from build123d import *
from build123d.topology import SkipClean

# Parameters (mm, degrees)
SKETCH_2_R               = 4.5
EXTRUDE_1_DEPTH          = 8
EXTRUDE_2_DEPTH          = 4
EXTRUDE_2_DEPTH_BACK     = 11.5
CUT_EXTRUDE_1_DEPTH      = 41.717122437
CUT_EXTRUDE_1_DEPTH_BACK = 41.717122437
CUT_EXTRUDE_2_DEPTH      = 41.717122437
CUT_EXTRUDE_2_DEPTH_BACK = 41.717122437
SKETCH_6_R               = 1
SKETCH_7_R               = 1.75
EXTRUDE_3_DEPTH          = 3
EXTRUDE_4_DEPTH          = 5
SKETCH_9_R               = 1
CUT_EXTRUDE_3_DEPTH      = 5
SKETCH_10_R              = 3.5
SKETCH_10_R_2            = 1
EXTRUDE_5_DEPTH          = 4


with BuildPart() as part:
    # Sketch 2 → Extrude 1 (new body)
    with BuildSketch(Plane.XY):
        with BuildLine():
            Line((-18.858561718, 18.044523082), (33.641438282, 18.044523082))
            ThreePointArc((33.641438282, 18.044523082), (34.348545063, 17.751629864), (34.641438282, 17.044523082))
            Line((34.641438282, 17.044523082), (34.641438282, 7.044523082))
            ThreePointArc((34.641438282, 7.044523082), (34.348545063, 6.337416301), (33.641438282, 6.044523082))
            Line((33.641438282, 6.044523082), (22.641438282, 6.044523082))
            ThreePointArc((22.641438282, 6.044523082), (19.105904376, 4.580056988), (17.641438282, 1.044523082))
            Line((17.641438282, 1.044523082), (17.641438282, -12.955476918))
            ThreePointArc((17.641438282, -12.955476918), (17.348545063, -13.662583699), (16.641438282, -13.955476918))
            Line((16.641438282, -13.955476918), (-9.858561718, -13.955476918))
            ThreePointArc((-9.858561718, -13.955476918), (-10.565668499, -13.662583699), (-10.858561718, -12.955476918))
            Line((-10.858561718, -12.955476918), (-10.858561718, 6.044523082))
            Line((-10.858561718, 6.044523082), (-17.858561718, 6.044523082))
            ThreePointArc((-17.858561718, 6.044523082), (-18.565668499, 6.337416301), (-18.858561718, 7.044523082))
            Line((-18.858561718, 7.044523082), (-18.858561718, 18.044523082))
        make_face()
        with Locations((-0.858561718, -3.955476918)):
            Circle(SKETCH_2_R, mode=Mode.SUBTRACT)
    extrude(amount=EXTRUDE_1_DEPTH)

    # Sketch 3 → Extrude 2 (add, two sides: drawn at the far end of the back side and taken through both)
    with SkipClean():  # the faces are left unmerged after this step: merging them gives an invalid solid
        with BuildSketch(Plane.XY.offset(8).offset(-EXTRUDE_2_DEPTH_BACK)):
            with BuildLine():
                Line((27.141438282, 14.544523082), (27.141438282, 18.044523082))
                Line((27.141438282, 18.044523082), (33.141438282, 18.044523082))
                Line((33.141438282, 18.044523082), (33.141438282, 14.544523082))
                ThreePointArc((33.141438282, 14.544523082), (30.141438282, 11.544523082), (27.141438282, 14.544523082))
            make_face()
            with BuildLine():
                Line((-0.358561718, 14.544523082), (-0.358561718, 18.044523082))
                Line((-0.358561718, 18.044523082), (-6.358561718, 18.044523082))
                Line((-6.358561718, 18.044523082), (-6.358561718, 14.544523082))
                ThreePointArc((-6.358561718, 14.544523082), (-3.358561718, 11.544523082), (-0.358561718, 14.544523082))
            make_face()
            with BuildLine():
                Line((-6.358561718, -10.455476918), (-6.358561718, -13.955476918))
                Line((-6.358561718, -13.955476918), (-0.358561718, -13.955476918))
                Line((-0.358561718, -13.955476918), (-0.358561718, -10.455476918))
                ThreePointArc((-0.358561718, -10.455476918), (-0.519059003, -9.487373446), (-0.983377938, -8.622855294))
                ThreePointArc((-0.983377938, -8.622855294), (-1.135599023, -8.491670945), (-1.327173883, -8.4310107))
                ThreePointArc((-1.327173883, -8.4310107), (-2.473967575, -8.155532145), (-3.509794913, -7.591541073))
                ThreePointArc((-3.509794913, -7.591541073), (-3.692643427, -7.508192328), (-3.893539312, -7.503562458))
                ThreePointArc((-3.893539312, -7.503562458), (-5.661270208, -8.532579726), (-6.358561718, -10.455476918))
            make_face()
        extrude(amount=EXTRUDE_2_DEPTH + EXTRUDE_2_DEPTH_BACK)
    add(part.part.scale(1), mode=Mode.REPLACE)  # the faces are merged on a copy

    # Sketch 5 → Cut-Extrude 1 (cut, two sides: drawn at the far end of the back side and taken through both)
    with BuildSketch(Plane.XY.offset(8).offset(-CUT_EXTRUDE_1_DEPTH_BACK)):
        with BuildLine():
            Line((8.520862779, 6.560547497), (2.520862779, 6.560547497))
            ThreePointArc((2.520862779, 6.560547497), (0.399542436, 5.681867841), (-0.479137221, 3.560547497))
            Line((-0.479137221, 3.560547497), (-0.479137221, -8.439452503))
            Line((-0.479137221, -8.439452503), (8.520862779, -8.439452503))
            ThreePointArc((8.520862779, -8.439452503), (10.642183123, -7.560772847), (11.520862779, -5.439452503))
            Line((11.520862779, -5.439452503), (11.520862779, 3.560547497))
            ThreePointArc((11.520862779, 3.560547497), (10.642183123, 5.681867841), (8.520862779, 6.560547497))
        make_face()
    extrude(amount=CUT_EXTRUDE_1_DEPTH + CUT_EXTRUDE_1_DEPTH_BACK, mode=Mode.SUBTRACT)

    # Sketch 6 → Cut-Extrude 2 (cut, two sides: drawn at the far end of the back side and taken through both)
    with BuildSketch(Plane.XY.offset(8).offset(-CUT_EXTRUDE_2_DEPTH_BACK)):
        with Locations((-3.358561718, 14.544523082)):
            Circle(SKETCH_6_R)
        with Locations((30.141438282, 14.544523082)):
            Circle(SKETCH_6_R)
        with Locations((-3.358561718, -10.455476918)):
            Circle(SKETCH_6_R)
    extrude(amount=CUT_EXTRUDE_2_DEPTH + CUT_EXTRUDE_2_DEPTH_BACK, mode=Mode.SUBTRACT)

    # Sketch 7 → Extrude 3 (add)
    with BuildSketch(Plane(origin=(0, 18.044523082, 0), x_dir=(1, 0, 0), z_dir=(0, 1, 0))):
        with BuildLine():
            Line((-31.858561718, 15.5), (95.141438282, 15.5))
            ThreePointArc((95.141438282, 15.5), (98.656156908, 7.014718626), (107.141438282, 3.5))
            Line((107.141438282, 3.5), (107.141438282, -56.5))
            ThreePointArc((107.141438282, -56.5), (98.656156908, -60.014718626), (95.141438282, -68.5))
            Line((95.141438282, -68.5), (-31.858561718, -68.5))
            ThreePointArc((-31.858561718, -68.5), (-35.373280344, -60.014718626), (-43.858561718, -56.5))
            Line((-43.858561718, -56.5), (-43.858561718, 3.5))
            ThreePointArc((-43.858561718, 3.5), (-35.373280344, 7.014718626), (-31.858561718, 15.5))
        make_face()
        with Locations(Location((-37.858561718, -26.5, 0), (0, 0, 180))):
            Circle(SKETCH_7_R, mode=Mode.SUBTRACT)
        with Locations(Location((-37.858561718, -50, 0), (0, 0, 180))):
            Circle(SKETCH_7_R, mode=Mode.SUBTRACT)
        with Locations(Location((-37.858561718, -3, 0), (0, 0, 180))):
            Circle(SKETCH_7_R, mode=Mode.SUBTRACT)
        with Locations((101.141438282, -50)):
            Circle(SKETCH_7_R, mode=Mode.SUBTRACT)
        with Locations((101.141438282, -26.5)):
            Circle(SKETCH_7_R, mode=Mode.SUBTRACT)
        with Locations((101.141438282, -3)):
            Circle(SKETCH_7_R, mode=Mode.SUBTRACT)
    extrude(amount=EXTRUDE_3_DEPTH)

    # Sketch 8 → Extrude 4 (add)
    with BuildSketch(Plane.XZ.offset(-18.044523082)):
        with BuildLine():
            Line((90.141438282, 31), (44.141438282, 31))
            ThreePointArc((44.141438282, 31), (42.72722472, 30.414213562), (42.141438282, 29))
            Line((42.141438282, 29), (42.141438282, 28))
            ThreePointArc((42.141438282, 28), (42.72722472, 26.585786438), (44.141438282, 26))
            Line((44.141438282, 26), (90.141438282, 26))
            ThreePointArc((90.141438282, 26), (91.555651845, 26.585786438), (92.141438282, 28))
            Line((92.141438282, 28), (92.141438282, 29))
            ThreePointArc((92.141438282, 29), (91.555651845, 30.414213562), (90.141438282, 31))
        make_face()
    extrude(amount=EXTRUDE_4_DEPTH)

    # Sketch 9 → Cut-Extrude 3 (cut)
    with BuildSketch(Plane.XZ.offset(-13.044523082)):
        with Locations((67.141438282, 28.5)):
            Circle(SKETCH_9_R)
        with Locations((72.141438282, 28.5)):
            Circle(SKETCH_9_R)
        with Locations((77.141438282, 28.5)):
            Circle(SKETCH_9_R)
        with Locations((82.141438282, 28.5)):
            Circle(SKETCH_9_R)
        with Locations((87.141438282, 28.5)):
            Circle(SKETCH_9_R)
        with Locations(Location((47.141438282, 28.5, 0), (0, 0, 180))):
            Circle(SKETCH_9_R)
        with Locations(Location((52.141438282, 28.5, 0), (0, 0, 180))):
            Circle(SKETCH_9_R)
        with Locations(Location((57.141438282, 28.5, 0), (0, 0, 180))):
            Circle(SKETCH_9_R)
        with Locations(Location((62.141438282, 28.5, 0), (0, 0, 180))):
            Circle(SKETCH_9_R)
    extrude(amount=-CUT_EXTRUDE_3_DEPTH, mode=Mode.SUBTRACT)

    # Sketch 10 → Extrude 5 (add)
    # profile 1 of 6: a face of its own
    with BuildSketch(Plane.XZ.offset(-18.044523082)):
        with Locations(Location((32.641438282, 55, 0), (0, 0, 180))):
            Circle(SKETCH_10_R)
        with Locations((32.641438282, 55)):
            Circle(SKETCH_10_R_2, mode=Mode.SUBTRACT)
    # profile 2 of 6: a face of its own
    with BuildSketch(Plane.XZ.offset(-18.044523082)):
        with Locations(Location((63.641438282, 39, 0), (0, 0, 180))):
            Circle(SKETCH_10_R)
        with Locations((63.641438282, 39)):
            Circle(SKETCH_10_R_2, mode=Mode.SUBTRACT)
    # profile 3 of 6: a face of its own
    with BuildSketch(Plane.XZ.offset(-18.044523082)):
        with Locations(Location((-28.258561718, 54, 0), (0, 0, 180))):
            Circle(SKETCH_10_R)
        with Locations((-28.258561718, 54)):
            Circle(SKETCH_10_R_2, mode=Mode.SUBTRACT)
    # profile 4 of 6: a face of its own
    with BuildSketch(Plane.XZ.offset(-18.044523082)):
        with Locations(Location((14.541438282, 54, 0), (0, 0, 180))):
            Circle(SKETCH_10_R)
        with Locations(Location((14.541438282, 54, 0), (0, 0, 180))):
            Circle(SKETCH_10_R_2, mode=Mode.SUBTRACT)
    # profile 5 of 6: a face of its own
    with BuildSketch(Plane.XZ.offset(-18.044523082)):
        with Locations(Location((14.541438282, 33, 0), (0, 0, 180))):
            Circle(SKETCH_10_R)
        with Locations((14.541438282, 33)):
            Circle(SKETCH_10_R_2, mode=Mode.SUBTRACT)
    # profile 6 of 6: a face of its own
    with BuildSketch(Plane.XZ.offset(-18.044523082)):
        with Locations(Location((-28.258561718, 33, 0), (0, 0, 180))):
            Circle(SKETCH_10_R)
        with Locations(Location((-28.258561718, 33, 0), (0, 0, 180))):
            Circle(SKETCH_10_R_2, mode=Mode.SUBTRACT)
    extrude(amount=EXTRUDE_5_DEPTH)


solid = part.part
Read the model definition and answer for the solid it produces. Units are mm, in the model's axes. A direction names the side the tool comes from. Round coordinates to 2 decimals unless told otherwise and drop trailing zeros. Write each loop counter-clockwise with the first axis right and the second up, starting at its lowest first coordinate (ties: lowest second). Pieces come first, ordered by that corner, then holes.
Q1. Find section B-B on y = -4. Determine the outline of the cut face in (x, z), and give its area (3 significant figures).
Values:
outline: (-10.86, 0) - (-5.36, 0) - (-5.36, 8) - (-10.86, 8) - close; (11.52, 0) - (17.64, 0) - (17.64, 8) - (11.52, 8) - close
area: 93.0 mm2
Q2. Flat-ended cylindrical pins translate along their axes: P1, Ø3, axis at x = 31, y = 14.5, coming from the +Z side; P2, Ø4, axis at x = -0.5, y = 15.5, coming from the +Z side; P3, Ø2.5, axis at x = -3.36, y = -10.46, coming from the -Z side; P4, Ø8, axis at y = 1, z = -7, coming from the -X side (3 decimals). Find the tip coordinate at first contact, or state that the pin passes through.
Values:
P1: stops at z = 58.5
P2: stops at z = 12
P3: stops at z = -3.5
P4: passes through
Q3. A tool of negligible diameter and unlimited length cuts with its end or side. For faces 1 (the face through (-3.425, 11.545, 9.972)), 2 (the face through (-27.8, 16.07, 50.53)), 3 (the face through (-6.359, -12, -2)), from which of +Z, -Z, +X, -X, +Y, -Y can it reach the whole face along a straight path? Write none if from no direction.
Values:
face 1: +Z
face 2: -Y
face 3: -Z, -X, -Y
Q4. Find section C-C on x = 19.5. Determine the outline of the cut face in (y, z), and give its area (3 significant figures).
Values:
outline: (4.93, 0) - (18.04, 0) - (18.04, -15.5) - (21.04, -15.5) - (21.04, 68.5) - (18.04, 68.5) - (18.04, 8) - (4.93, 8) - close
area: 357 mm2
Q5. The mould has two halves that part along Z. Classify faces 4 (the face through (33, 20, 68.5)), 5 (the face through (4, -13.955, 4)), 6 (the face through (102.81, 19.52, 2.47)), 7 (the face through (31, 20, -15.5)): released by +Z, released by -Z, zero draft, split by the parting line, or undercut.
Values:
face 4: released by +Z
face 5: zero draft
face 6: undercut
face 7: released by -Z
Q6. Find section A-A on z = 3. State how many separate pieces and enclosed holes the cut face has, and give its area (3 significant figures).
Values:
separate pieces: 3
enclosed holes: 4
area: 1,430 mm2
Q7. Straight lines are drawn through the part: line 1 (Y direction, x = 80, z = 63); line 2 (Z direction, x = 48.5, y = 18); line 3 (Z direction, x = 4, y = -11). For each, find the intervals that lie inside material, in ascending order.
Values:
line 1: y = 18.04 to 21.04
line 2: z = 26 to 31
line 3: z = 0 to 8
Q8. Find section D-D on z = -10. Determine the outline of the cut face in (x, y), and give its area (3 significant figures).
Values:
outline: (-33.19, 18.04) - (96.48, 18.04) - (96.48, 21.04) - (-33.19, 21.04) - close
area: 389 mm2
